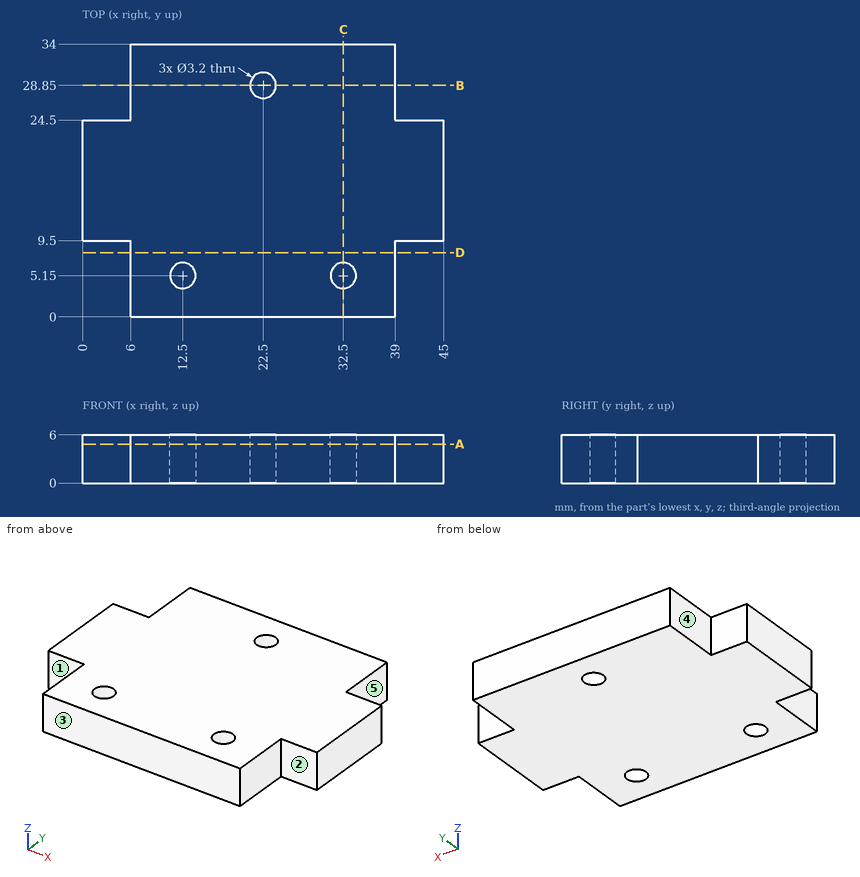
For this review, use the dimensioned drawing (mm, ordinates from the lowest corner) and the shaded views. A direction names the side the tool comes from. Coordinates: 2 decimals unless noted, no trailing zeros. Loops run counter-clockwise (first coordinate to the right, second up) from the corner with the lowest first, then second, coordinate; pieces in that order, holes last. Notation, with made-up numbers: (32, 39) - (50, 39) arc R20 ccw to (50, 48) - close; hole circle Ø3 at (1, 3.5). An arc over 180 degrees is marked (long way). Use CSV: the item, a comma, the result in double quotes. Start each with the question number.
1) Consider section D-D on y = 8. Write out the cut boundary in (x, z).
2) Consider section C-C on x = 32.5. Write out the cut boundary in (y, z).
3) For pin 1 Ø1.8 at (y, z) = (27.5, 3.5) entering from +X; pin 2 Ø3 at (x, z) = (2, 4.5) entering from -Y; pin 3 Ø3 at (x, z) = (41.5, 3) entering from +Y, all flat-tipped, find the tip position at first contact; note any pin that passes through.
4) Tool access review of the marked faces 1, 2, 3, 4 and 5: name each direction out of +Z, -Z, +X, -X, +Y, -Y from which nothing blocks a thin tool from reaching the whole face with its end or side.
5) Consider section B-B on y = 28.85. Write out the cut boundary in (x, z).
6) Wall thickness on L1, parallel to Y at x = 22.5, z = 4.4; L2, parallel to Y at x = 12.5, z = 1; L3, parallel to X at y = 2.5, z = 3.15: over which ranges is each line inside the solid? List them lowest first. Write a range as from..to.
7) Consider section A-A on z = 4.85. Write out the cut boundary in (x, y), then the cut area to 3 significant figures.
Geometry says:
1,outline,"(6, 0) - (39, 0) - (39, 6) - (6, 6) - close"
2,outline,"(0, 0) - (3.55, 0) - (3.55, 6) - (0, 6) - close; (6.75, 0) - (34, 0) - (34, 6) - (6.75, 6) - close"
3,pin 1,"x = 39"
3,pin 2,"y = 9.5"
3,pin 3,"y = 24.5"
4,face 1,"+Z, -Z, -X, -Y"
4,face 2,"+Z, -Z, +X, -Y"
4,face 3,"+Z, -Z, +X, -X, -Y"
4,face 4,"+Z, -Z, -X, +Y"
4,face 5,"+Z, -Z, +X, +Y"
5,outline,"(6, 0) - (20.9, 0) - (20.9, 6) - (6, 6) - close; (24.1, 0) - (39, 0) - (39, 6) - (24.1, 6) - close"
6,L1,"0..27.25, 30.45..34"
6,L2,"0..3.55, 6.75..34"
6,L3,"6..39"
7,outline,"(0, 9.5) - (6, 9.5) - (6, 0) - (39, 0) - (39, 9.5) - (45, 9.5) - (45, 24.5) - (39, 24.5) - (39, 34) - (6, 34) - (6, 24.5) - (0, 24.5) - close; hole circle Ø3.2 at (12.5, 5.15); hole circle Ø3.2 at (22.5, 28.85); hole circle Ø3.2 at (32.5, 5.15)"
7,area,"1,280 mm^2"
